from build123d import *

# Parameters (mm, degrees)
SKETCH1_R           = 88.9
BOSS_EXTRUDE1_DEPTH = 50
SKETCH2_R           = 82.55
CUT_EXTRUDE4_DEPTH  = 74
SKETCH12_R          = 22.5
CUT_EXTRUDE5_DEPTH  = 115.64
SKETCH13_R          = 22.5
CUT_EXTRUDE6_DEPTH  = 115.64
SKETCH14_R          = 22.5
CUT_EXTRUDE7_DEPTH  = 99.64
SKETCH15_R          = 22.5
CUT_EXTRUDE8_DEPTH  = 137.64


with BuildPart() as part:
    # Sketch1 → Boss-Extrude1 (new body)
    with BuildSketch(Plane(origin=(0, 0, 0), x_dir=(1, 0, 0), z_dir=(0, 1, 0))):
        Circle(SKETCH1_R)
    extrude(amount=BOSS_EXTRUDE1_DEPTH)

    # Sketch2 → Cut-Extrude4 (cut)
    with BuildSketch(Plane(origin=(0, 0, 0), x_dir=(1, 0, 0), z_dir=(0, 1, 0))):
        Circle(SKETCH2_R)
    extrude(amount=CUT_EXTRUDE4_DEPTH, mode=Mode.SUBTRACT)

    # Sketch12 → Cut-Extrude5 (cut)
    with BuildSketch(Plane(origin=(0, 0, 0), x_dir=(0, 0, -1), z_dir=(1, 0, 0))):
        with Locations((0, 24.336091646)):
            Circle(SKETCH12_R)
    extrude(amount=-CUT_EXTRUDE5_DEPTH, mode=Mode.SUBTRACT)

    # Sketch13 → Cut-Extrude6 (cut)
    with BuildSketch(Plane.XY):
        with Locations((0, 25.450721797)):
            Circle(SKETCH13_R)
    extrude(amount=-CUT_EXTRUDE6_DEPTH, mode=Mode.SUBTRACT)

    # Sketch14 → Cut-Extrude7 (cut)
    with BuildSketch(Plane(origin=(0, 0, 0), x_dir=(0, 0, -1), z_dir=(1, 0, 0))):
        with Locations((0, 24.521863338)):
            Circle(SKETCH14_R)
    extrude(amount=CUT_EXTRUDE7_DEPTH, mode=Mode.SUBTRACT)

    # Sketch15 → Cut-Extrude8 (cut)
    with BuildSketch(Plane.XY):
        with Locations((0, 25.450721797)):
            Circle(SKETCH15_R)
    extrude(amount=CUT_EXTRUDE8_DEPTH, mode=Mode.SUBTRACT)


solid = part.part
Geometry check sheet. Reference: the model listing, model coordinates, mm. Give positions to 0.01 mm unless a question says otherwise; leave off trailing zeros. Order: outer loops, then holes, each group sorted by start corner. A loop starts at its lowest first (then second) coordinate and runs counter-clockwise, first axis right, second up. Notation, with made-up numbers: M 70,56.25 L 80,56.25 A19 ccw 80,81.25 Z; hole C -9.75,33.5 d9. An arc over 180 degrees is marked long. Use a Markdown table: item, result.
Item 1: Section check A-A (z = 0). Record the cut outline in (x, y), and give its area (3 significant figures).
Answers follow:
| item | result |
|---|---|
| outline | M -88.9,0 L -82.55,0 L -82.55,1.84 L -88.9,1.84 Z; M -88.9,46.84 L -82.55,46.84 L -82.55,50 L -88.9,50 Z; M 82.55,0 L 88.9,0 L 88.9,2.02 L 82.55,2.02 Z; M 82.55,47.02 L 88.9,47.02 L 88.9,50 L 82.55,50 Z |
| area | 63.5 mm2 |
Item 2: Section check B-B (x = 0). Record the cut outline in (y, z).
Answers follow:
| item | result |
|---|---|
| outline | M 0,-88.9 L 2.95,-88.9 L 2.95,-82.55 L 0,-82.55 Z; M 0,82.55 L 2.95,82.55 L 2.95,88.9 L 0,88.9 Z; M 47.95,-88.9 L 50,-88.9 L 50,-82.55 L 47.95,-82.55 Z; M 47.95,82.55 L 50,82.55 L 50,88.9 L 47.95,88.9 Z |
Item 3: Draft check along Y on faces 1 (the flat face through (26, 0, 79)), 2 (the flat face through (26, 50, 79)), 3 (the cylindrical face through (84.1, 43.49, -12.1)), 4 (the cylindrical face through (-84.096, 43.308, -12.096)). Enter one of: +Y half, -Y half, draft (parallel to the pull), parting line (faces both ways), or undercut.
Answers follow:
| item | result |
|---|---|
| face 1 | -Y half |
| face 2 | +Y half |
| face 3 | undercut |
| face 4 | undercut |
Item 4: Material ranges on line 1 along Y through (x, z) = (-85, 0); line 2 along Y through (x, z) = (0, -83.75); line 3 along X through (y, z) = (11, -22), recorded low to high.
Answers follow:
| item | result |
|---|---|
| line 1 | y = 0 to 1.84, 46.84 to 50 |
| line 2 | y = 0 to 2.95, 47.95 to 50 |
| line 3 | x = -86.13 to -79.56, 79.56 to 86.13 |
Item 5: Depth check by flat-ended pin: P1, Ø1.5, axis at x = -51.5, y = 17, coming from the +Z side; P2, Ø12, axis at y = 44, z = 58.5, coming from the +X side; P3, Ø1.5, axis at y = 19, z = 27.5, coming from the +X side. Enter the tip coordinate at first touch or a pass-through.
Answers follow:
| item | result |
|---|---|
| P1 | stops at z = 72.99 |
| P2 | stops at x = 71.74 |
| P3 | stops at x = 84.78 |
Item 6: Section check C-C (x = 60.5). Record the cut outline in (y, z), and give its area (3 significant figures).
Answers follow:
| item | result |
|---|---|
| outline | M 0,-65.14 L 50,-65.14 L 50,-56.16 L 0,-56.16 Z; M 0,56.16 L 50,56.16 L 50,65.14 L 0,65.14 Z |
| area | 898 mm2 |
Item 7: Section check D-D (z = -50.5). Record the cut outline in (x, y).
Answers follow:
| item | result |
|---|---|
| outline | M -73.16,0 L -65.3,0 L -65.3,50 L -73.16,50 Z; M 65.3,0 L 73.16,0 L 73.16,50 L 65.3,50 Z |
